Autodesk Inventor part; units mm, degrees
ref_plane "A4_XY" through (455, 0, 0) normal (0, 1, 0) x (1, 0, 0)
ref_plane "A4_YZ" through (455, 0, 0) normal (1, 0, 0) x (0, 0, -1)
ref_plane "A4_ZX" through (455, 0, 0) normal (0, 0, -1) x (0, 1, 0)
sketch "Sketch_9" plane through (0, 0, 0) normal (0, 0, 1) x (1, 0, 0)
  line L0 (207.5, 0) -> (-54, 0)
  line L1 (-54, 0) -> (-54, 5.233)
  line L2 (-54, 5.233) -> (-53.233, 6)
  line L3 (-53.233, 6) -> (-32.767, 6)
  line L4 (-32.767, 6) -> (-32, 5.233)
  line L5 (-32, 5.233) -> (-32, 5.2)
  line L6 (-32, 5.2) -> (-30, 5.2)
  line L7 (-30, 5.2) -> (-30, 7)
  line L8 (-30, 7) -> (-28.2679, 8)
  line L9 (-28.2679, 8) -> (197.5, 8)
  line L10 (197.5, 8) -> (197.5, 20)
  line L11 (197.5, 20) -> (207.5, 20)
  line L12 (207.5, 20) -> (207.5, 0)
  line L13 (207.5, 0) -> (-54, 0)
revolve "Revolution1" add sketch "Sketch_9" angle 360 about axis through (207.5, 0, 0) along (1, 0, 0)
thread "Thread1"
sketch "Sketch_4" plane through (-30, 0, 0) normal (1, 0, 0) x (0, 0, -1)
  line L0 (-15, -11.5) -> (15, -11.5)
  line L1 (15, -11.5) -> (15, 11.5)
  line L2 (15, 11.5) -> (-15, 11.5)
  line L3 (-15, 11.5) -> (-15, -11.5)
  line L4 (-10, 6.5) -> (-10, -6.5)
  line L5 (-10, -6.5) -> (10, -6.5)
  line L6 (10, -6.5) -> (10, 6.5)
  line L7 (10, 6.5) -> (-10, 6.5)
extrude "Extrusion1" cut sketch "Sketch_4" along normal blind 6.5
ref_plane "A4_XY" through (455, 0, 0) normal (0, 1, 0) x (1, 0, 0)
ref_plane "A4_YZ" through (455, 0, 0) normal (1, 0, 0) x (0, 0, -1)
ref_plane "A4_ZX" through (455, 0, 0) normal (0, 0, -1) x (0, 1, 0)
ref_plane "ROD_BODY_XY" through (0, 0, 0) normal (1, 0, 0) x (0, 0, -1)
ref_plane "ROD_BODY_YZ" through (0, 0, 0) normal (0, 0, -1) x (0, 1, 0)
ref_plane "ROD_BODY_ZX" through (0, 0, 0) normal (0, 1, 0) x (1, 0, 0)
ref_plane "ROD_NUT_XY" through (-54, 0, 0) normal (-1, 0, 0) x (0, 0, -1)
ref_plane "ROD_NUT_YZ" through (-54, 0, 0) normal (0, 0, -1) x (0, -1, 0)
ref_plane "ROD_NUT_ZX" through (-54, 0, 0) normal (0, -1, 0) x (-1, 0, 0)
properties part number "CP96S40-160_ROD" material "Stainless Steel, Polished"
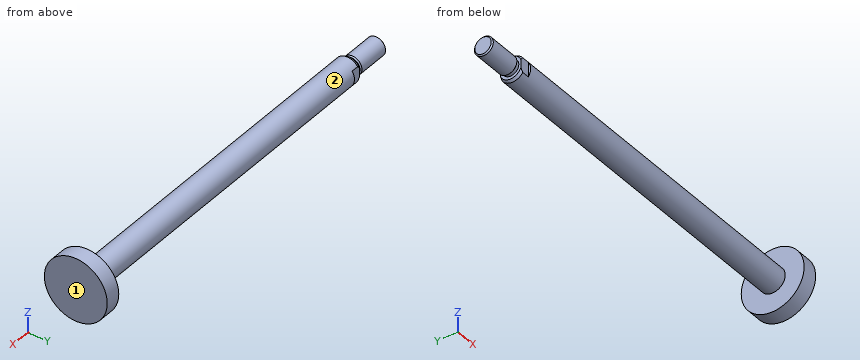
Verification items for the finished model (mm, model axes). Face numbers are marked on the shaded views. A direction names the side the tool comes from. Round coordinates to 2 decimals unless told otherwise and drop trailing zeros. Order: outer loops, then holes, each group sorted by start corner. A loop starts at its lowest first (then second) coordinate and runs counter-clockwise, first axis right, second up. Notation, with made-up numbers: (51, 84.5) - (102, 84.5) arc R18 cw to (102, 94.5) - close; hole circle Ø5 at (14, -28). An arc over 180 degrees is marked (long way). Use CSV: the item, a comma, the result in double quotes. Start each with the question number.
1) Section check D-D, the plane z = 15. Record the cut outline in (x, y), plus the area to 3 significant figures.
2) Access from +Z, -Z, +X, -X, +Y, -Y to the whole of each face (thin tool, end or side, straight path). Record for the marked faces 1 and 2.
3) Section check C-C, the plane x = 185. Record the cut outline in (y, z).
4) Thickness scan on L1, parallel to X at y = 0.5, z = -16.5; L2, parallel to Z at x = 193, y = 0; L3, parallel to Y at x = 113.5, z = -0.5. Record the ranges inside material, lowest first.
5) Go/stop test with flat-tipped pins: P1, Ø6, axis at x = -11, z = -13, coming from the -Y side; P2, Ø5, axis at x = 135.5, y = -7, coming from the -Z side; P3, Ø5, axis at x = -27, z = 0.5, coming from the +Y side; P4, Ø10, axis at x = 116.5, y = -2, coming from the +Z side. Record where each tip stops, or that it passes through.
Answers:
1,outline,"(197.5, -13.23) - (207.5, -13.23) - (207.5, 13.23) - (197.5, 13.23) - close"
1,area,"265 mm²"
2,face 1,"+Z, -Z, +X, +Y, -Y"
2,face 2,"-X"
3,outline,"circle Ø16 at (0, 0)"
4,L1,"x = 197.5 to 207.5"
4,L2,"z = -8 to 8"
4,L3,"y = -7.98 to 7.98"
5,P1,"passes through"
5,P2,"stops at z = -6.61"
5,P3,"stops at y = 6.5"
5,P4,"stops at z = 8"
